Geometry check sheet. Reference: drawing and pictorial views, mm from the part's lowest x, y, z. A direction names the side the tool comes from. Give positions to 0.01 mm unless a question says otherwise; leave off trailing zeros. Write each loop counter-clockwise with the first axis right and the second up, starting at its lowest first coordinate (ties: lowest second). Pieces come first, ordered by that corner, then holes.
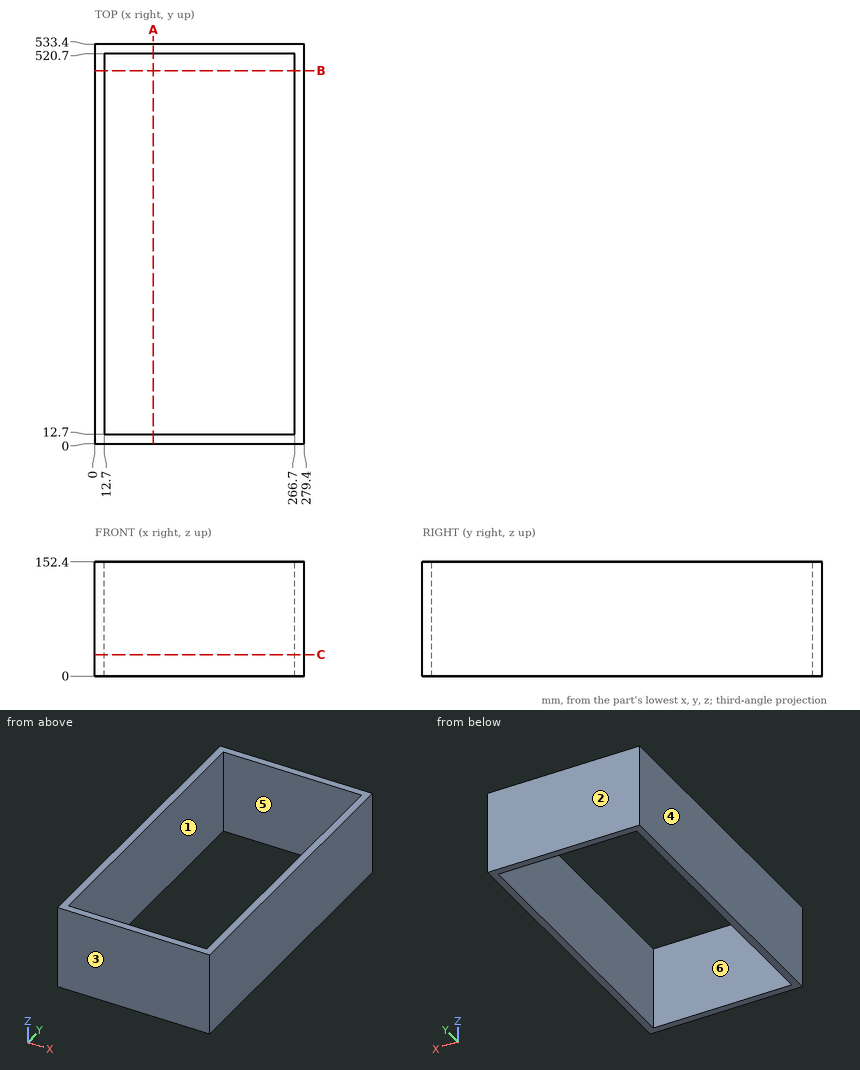
Item 1: Scan lines: line 1 along Y through (x, z) = (232.5, 90); line 2 along X through (y, z) = (420, 53.5). Record each from-to range of solid material in increasing order.
Answer key:
line 1: y = 0 to 12.7, 520.7 to 533.4
line 2: x = 0 to 12.7, 266.7 to 279.4
Item 2: Sectioned sample at B-B on y = 498. Record the cut outline in (x, z), then the cut area to 3 significant figures.
Answer key:
outline: (0, 0) - (12.7, 0) - (12.7, 152.4) - (0, 152.4) - close; (266.7, 0) - (279.4, 0) - (279.4, 152.4) - (266.7, 152.4) - close
area: 3,870 mm2
Item 3: Sectioned sample at C-C on z = 28.5. Record the cut outline in (x, y).
Answer key:
outline: (0, 0) - (279.4, 0) - (279.4, 533.4) - (0, 533.4) - close; hole (12.7, 12.7) - (266.7, 12.7) - (266.7, 520.7) - (12.7, 520.7) - close
Item 4: Release check for a two-part mould opening along X. For the marked faces 3, 4, 5 and 6 record: released by +X, released by -X, zero draft, split by the parting line, or undercut.
Answer key:
face 3: zero draft
face 4: released by -X
face 5: undercut
face 6: undercut
Item 5: Set-up check for the marked faces 1 and 2: record each of +Z, -Z, +X, -X, +Y, -Y from which the full face is reachable in a straight line by a thin tool's end or side.
Answer key:
face 1: +Z, -Z
face 2: +Z, -Z, +X, -X, +Y
Item 6: Sectioned sample at A-A on x = 78. Record the cut outline in (y, z).
Answer key:
outline: (0, 0) - (12.7, 0) - (12.7, 152.4) - (0, 152.4) - close; (520.7, 0) - (533.4, 0) - (533.4, 152.4) - (520.7, 152.4) - close
